Geometry check sheet. Reference: the model listing, model coordinates, mm. Coordinates: 2 decimals unless noted, no trailing zeros. Loops run counter-clockwise (first coordinate to the right, second up) from the corner with the lowest first, then second, coordinate; pieces in that order, holes last.
from build123d import *

# Parameters (mm, degrees)
SKETCH1_W           = 810
SKETCH1_H           = 410
BOSS_EXTRUDE1_DEPTH = 15
SHELL1_T            = -2
SKETCH2_W           = 790
SKETCH2_H           = 390
CUT_EXTRUDE1_DEPTH  = 15


with BuildPart() as part:
    # Sketch1 → Boss-Extrude1 (new body)
    with BuildSketch(Plane(origin=(0, 0, 0), x_dir=(1, 0, 0), z_dir=(0, 1, 0))):
        with Locations((405, 205)):
            Rectangle(SKETCH1_W, SKETCH1_H)
    extrude(amount=BOSS_EXTRUDE1_DEPTH)

    # Shell1
    shell1_openings = [part.faces().sort_by_distance(p)[0] for p in [
        (405, 0, -205),
    ]]
    offset(amount=SHELL1_T, openings=shell1_openings, kind=Kind.INTERSECTION)

    # Sketch2 → Cut-Extrude1 (cut)
    with BuildSketch(Plane(origin=(0, 15, 0), x_dir=(1, 0, 0), z_dir=(0, 1, 0))):
        with Locations((405, 205)):
            Rectangle(SKETCH2_W, SKETCH2_H)
    extrude(amount=-CUT_EXTRUDE1_DEPTH, mode=Mode.SUBTRACT)


solid = part.part
(1) Draft check along Y on faces 1 (the flat face through (399, 7, 0)), 2 (the flat face through (403, 13, -401)), 3 (the flat face through (403, 15, -9)). Enter one of: +Y half, -Y half, draft (parallel to the pull), parting line (faces both ways), or undercut.
Findings:
face 1: draft
face 2: -Y half
face 3: +Y half
(2) Sectioned sample at A-A on z = -289.5. Record the cut outline in (x, y).
Findings:
outline: (0, 0) - (2, 0) - (2, 13) - (10, 13) - (10, 15) - (0, 15) - close; (800, 13) - (808, 13) - (808, 0) - (810, 0) - (810, 15) - (800, 15) - close
(3) Sectioned sample at C-C on x = 314. Record the cut outline in (y, z).
Findings:
outline: (0, -410) - (15, -410) - (15, -400) - (13, -400) - (13, -408) - (0, -408) - close; (0, -2) - (13, -2) - (13, -10) - (15, -10) - (15, 0) - (0, 0) - close
(4) Sectioned sample at B-B on y = 6. Record the cut outline in (x, z).
Findings:
outline: (0, -410) - (810, -410) - (810, 0) - (0, 0) - close; hole (2, -408) - (808, -408) - (808, -2) - (2, -2) - close
(5) Scan lines: L1, parallel to Z at x = 747.5, y = 8; L2, parallel to X at y = 5, z = -96; L3, parallel to Z at x = 173, y = 14.25. Record each from-to range of solid material in increasing order.
Findings:
L1: z = -410 to -408, -2 to 0
L2: x = 0 to 2, 808 to 810
L3: z = -410 to -400, -10 to 0
